from build123d import *

# Parameters (mm, degrees)
SKETCH1_W           = 150
SKETCH1_H           = 30
BOSS_EXTRUDE1_DEPTH = 4
FILLET1_R           = 5


with BuildPart() as part:
    # Sketch1 → Boss-Extrude1 (new body)
    with BuildSketch(Plane(origin=(0, 0, 0), x_dir=(1, 0, 0), z_dir=(0, 1, 0))):
        Rectangle(SKETCH1_W, SKETCH1_H)
        with BuildLine():
            Line((-62.5, 2.75), (62.5, 2.75))
            ThreePointArc((62.5, 2.75), (65.25, 0), (62.5, -2.75))
            Line((62.5, -2.75), (-62.5, -2.75))
            ThreePointArc((-62.5, -2.75), (-65.25, 0), (-62.5, 2.75))
        make_face(mode=Mode.SUBTRACT)
    extrude(amount=BOSS_EXTRUDE1_DEPTH)

    # Fillet1
    fillet1_edges = [part.edges().sort_by_distance(p)[0] for p in [
        (75, 2, 15),
        (-75, 2, 15),
        (-75, 2, -15),
        (75, 2, -15),
    ]]
    fillet(fillet1_edges, radius=FILLET1_R)


solid = part.part
Input: part model. Units: mm. Frame: model coordinates. A direction names the side the tool comes from. Coordinates: 2 decimals unless noted, no trailing zeros. Loops run counter-clockwise (first coordinate to the right, second up) from the corner with the lowest first, then second, coordinate; pieces in that order, holes last.
(1) Section B-B on y = 1.9. Return the cut outline in (x, z), then the cut area to 3 significant figures.
(2) Set-up query: faces 4 (the face through (-1, 2, -15)), 5 (the face through (1, 2, 2.75)). Return all of +Z, -Z, +X, -X, +Y, -Y with unobstructed straight access to the full face (end or side cutting, diameter ignored); none if empty.
(3) Section A-A on x = 5.5. Return the cut outline in (y, z), then the cut area to 3 significant figures.
(4) Pull-direction query (X, two-part tool) for faces 1 (the face through (-1, 2, -2.75)), 2 (the face through (73, 2, -14)), 3 (the face through (-1, 0, -4)); classes: released by +X, released by -X, zero draft, split by the parting line, or undercut.
(5) Material intervals for probe 1 along Z at (x, y) = (-1.5, 1.45); probe 2 along X at (y, z) = (0.65, -1.25), sorted ascending.
(6) First-contact query: pin 1 Ø1 at (y, z) = (3.5, 11.5) entering from -X; pin 2 Ø1 at (x, z) = (-55.5, -1) entering from +Y. Flat tips, straight axial feed; report the tip coordinate or a pass-through.
(7) Section C-C on z = 0. Return the cut outline in (x, y).
Data:
1. outline: (-75, -10) arc R5 ccw to (-70, -15) - (70, -15) arc R5 ccw to (75, -10) - (75, 10) arc R5 ccw to (70, 15) - (-70, 15) arc R5 ccw to (-75, 10) - close; hole (-62.5, -2.75) - (62.5, -2.75) arc R2.75 ccw to (62.5, 2.75) - (-62.5, 2.75) arc R2.75 ccw to start
1. area: 3,770 mm2
2. face 4: -Z, +X, -X, +Y, -Y
2. face 5: +Y, -Y
3. outline: (0, -15) - (4, -15) - (4, -2.75) - (0, -2.75) - close; (0, 2.75) - (4, 2.75) - (4, 15) - (0, 15) - close
3. area: 98.0 mm2
4. face 1: undercut
4. face 2: released by +X
4. face 3: zero draft
5. probe 1: z = -15 to -2.75, 2.75 to 15
5. probe 2: x = -75 to -64.95, 64.95 to 75
6. pin 1: stops at x = -74.9
6. pin 2: passes through
7. outline: (-75, 0) - (-65.25, 0) - (-65.25, 4) - (-75, 4) - close; (65.25, 0) - (75, 0) - (75, 4) - (65.25, 4) - close
